Read the model definition and answer for the solid it produces. Units are mm, in the model's axes. Face numbers are marked on the shaded views. Coordinates: 2 decimals unless noted, no trailing zeros. Order: outer loops, then holes, each group sorted by start corner. A loop starts at its lowest first (then second) coordinate and runs counter-clockwise, first axis right, second up.
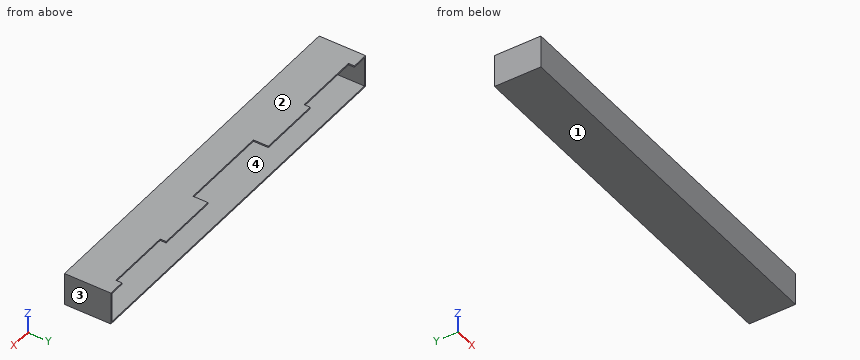
from build123d import *

# Parameters (mm, degrees)
BOSS_EXTRUDE1_DEPTH = 69.85
SKETCH3_W           = 796.798
SKETCH3_H           = 63.5
CUT_EXTRUDE1_DEPTH  = 95.25
CUT_EXTRUDE3_DEPTH  = 3.175


with BuildPart() as part:
    # Sketch2 → Boss-Extrude1 (new body)
    with BuildSketch(Plane.XY):
        Polygon((90.424, 0), (357.124, 0), (401.447, 0), (401.447, 98.425), (-401.701, 98.425), (-401.701, 0), (-366.776, 0), (-227.076, 0), (-100.076, 0), align=None)
    extrude(amount=BOSS_EXTRUDE1_DEPTH)

    # Sketch3 → Cut-Extrude1 (cut)
    with BuildSketch(Plane(origin=(0, 98.425, 0), x_dir=(1, 0, 0), z_dir=(0, 1, 0))):
        with Locations((-0.0635, -34.925)):
            Rectangle(SKETCH3_W, SKETCH3_H)
    extrude(amount=-CUT_EXTRUDE1_DEPTH, mode=Mode.SUBTRACT)

    # Sketch4 → Cut-Extrude3 (cut)
    with BuildSketch(Plane.XY.offset(69.85)):
        Polygon((-366.776, 98.425), (-366.776, 85.725), (-227.076, 85.725), (-227.076, 189.981198682), (-227.076, 207.999074197), (-95.25, 207.999074197), (-95.25, 98.425), (-95.25, 66.675), (95.25, 66.675), (95.25, 98.425), (95.25, 207.999074197), (227.076, 207.999074197), (227.076, 98.425), (227.076, 85.725), (366.776, 85.725), (366.776, 98.425), (366.776, 207.999074197), (366.776, 225.818081793), (-366.776, 225.818081793), (-366.776, 207.999074197), align=None)
    extrude(amount=-CUT_EXTRUDE3_DEPTH, mode=Mode.SUBTRACT)


solid = part.part
Q1. Determine the mould class of the marked faces 1, 2, 3 and 4 for opening direction Z: +Z half, -Z half, draft (parallel to the pull), parting line (faces both ways), or undercut.
Q2. Each of these flat-tipped pins is pushed along its axis until it touches: P1, Ø6, axis at x = -238, z = 57.5, coming from the +Y side (3 decimals); P2, Ø1.6, axis at x = -295, z = 68, coming from the +Y side (3 decimals); P3, Ø3.5, axis at x = -38, z = 68.5, coming from the +Y side (3 decimals). Where does it stop, or does it pass through?
Q3. The part is cut by section B-B, the plane x = -255.5. Determine the outline of the cut face in (y, z) (3 decimals).
Q4. The part is cut by section D-D, the plane z = 15. Determine the outline of the cut face in (x, y) (1 decimal), then the cut area to 3 significant figures.
Q5. Straight lines are drawn through the part: L1, parallel to Z at x = 151.5, y = 85 (3 decimals); L2, parallel to X at y = 78.5, z = 21; L3, parallel to Y at x = -49.5, z = 40.5 (3 decimals). For each, find the intervals that lie inside material, in ascending order.
Computed values:
1. face 1: -Z half
1. face 2: +Z half
1. face 3: draft
1. face 4: undercut
2. P1: stops at y = 3.175
2. P2: stops at y = 85.725
2. P3: stops at y = 66.675
3. outline: (0, 0) - (98.425, 0) - (98.425, 3.175) - (3.175, 3.175) - (3.175, 66.675) - (85.725, 66.675) - (85.725, 69.85) - (0, 69.85) - close
4. outline: (-401.7, 0) - (401.4, 0) - (401.4, 98.4) - (398.3, 98.4) - (398.3, 3.2) - (-398.5, 3.2) - (-398.5, 98.4) - (-401.7, 98.4) - close
4. area: 3,150 mm2
5. L1: z = 0 to 3.175, 66.675 to 69.85
5. L2: x = -401.7 to -398.46, 398.34 to 401.45
5. L3: y = 0 to 3.175
